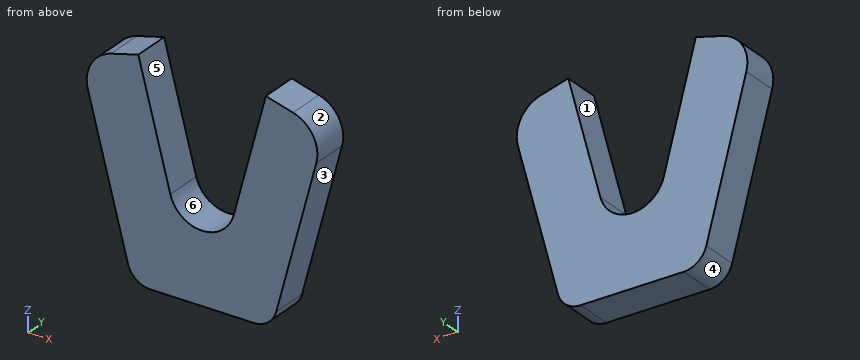
from build123d import *

# Parameters (mm, degrees)
F1_DEPTH = 25.4


with BuildPart() as f1:
    # F0 (on Front) → F1 (new body)
    with BuildSketch(Plane.XZ):
        with BuildLine():
            ThreePointArc((-50.266767, -58.054928), (-44.600918, -66.560398), (-34.925, -69.85))
            Line((-34.925, -69.85), (34.925, -69.85))
            ThreePointArc((34.925, -69.85), (44.600918, -66.560398), (50.266767, -58.054928))
            Line((50.266767, -58.054928), (77.358474, 43.8181))
            ThreePointArc((77.358474, 43.8181), (75.106497, 60.678651), (61.5919, 71.008474))
            Line((61.5919, 71.008474), (43.183091, 75.904039))
            Line((43.183091, 75.904039), (21.478474, -5.7119))
            ThreePointArc((21.478474, -5.7119), (0, -22.225), (-21.478474, -5.7119))
            Line((-21.478474, -5.7119), (-43.183091, 75.904039))
            Line((-43.183091, 75.904039), (-61.5919, 71.008474))
            ThreePointArc((-61.5919, 71.008474), (-75.106497, 60.678651), (-77.358474, 43.8181))
            Line((-77.358474, 43.8181), (-50.266767, -58.054928))
        make_face()
    extrude(amount=F1_DEPTH)


solid = f1.part
Work out the finished part from the listing and answer in its coordinate system (mm). Face numbers are marked on the shaded views. A direction names the side the tool comes from. Give positions to 0.01 mm unless a question says otherwise; leave off trailing zeros. Write each loop counter-clockwise with the first axis right and the second up, starting at its lowest first coordinate (ties: lowest second). Pieces come first, ordered by that corner, then holes. Notation, with made-up numbers: (48.5, -36) - (64.5, -36) arc R33 cw to (64.5, -8) - close; hole circle Ø9 at (-36, 58.5). An arc over 180 degrees is marked (long way). One line per item, written item: value. Start each with the question number.
1. Consider probe 1 along X at (y, z) = (-22.5, 33.5); probe 2 along X at (y, z) = (-18.75, 62); probe 3 along Z at (x, y) = (6, -9.25). Determine where each line is inside the solid, lowest interval first.
2. For the marked faces 1 and 2, determine the directions among +Z, -Z, +X, -X, +Y, -Y from which every point of the face is accessible in a straight line to the end or side of a thin tool.
3. Find section D-D (z = 26.5). Write down the section's boundary in (x, y).
4. Find section B-B (z = -17). Write down the section's boundary in (x, y).
5. Find section A-A (y = -3.5). Write down the section's boundary in (x, z) (3 decimals).
6. For a pull along X with two mould halves and no side action, classify the marked faces 3, 4, 5 and 6 as +X half, -X half, draft (parallel to the pull), parting line (faces both ways), or undercut.
7. Find section C-C (x = -4.5). Write down the section's boundary in (y, z), then the cut area to 3 significant figures.
8. Given pin 1 (3 mm diameter, centred on x = -17.5, y = -15, fed in from +Z); pin 2 (4 mm diameter, centred on y = -20.5, z = -31, fed in from +X), each flat-ended and moving along its own axis, determine where each tip first touches the part or whether it passes through.
Geometry results:
1. probe 1: -74.61 to -31.91, 31.91 to 74.61
1. probe 2: -74.28 to -39.49, 39.49 to 74.28
1. probe 3: -69.85 to -21.4
2. face 1: +Z, +Y, -Y
2. face 2: +X, +Y, -Y
3. outline: (-72.75, -25.4) - (-30.04, -25.4) - (-30.04, 0) - (-72.75, 0) - close; (30.04, -25.4) - (72.75, -25.4) - (72.75, 0) - (30.04, 0) - close
4. outline: (-61.18, -25.4) - (-14.32, -25.4) - (-14.32, 0) - (-61.18, 0) - close; (14.32, -25.4) - (61.18, -25.4) - (61.18, 0) - (14.32, 0) - close
5. outline: (-77.358, 43.818) - (-50.267, -58.055) arc R15.875 ccw to (-34.925, -69.85) - (34.925, -69.85) arc R15.875 ccw to (50.267, -58.055) - (77.358, 43.818) arc R22.225 ccw to (61.592, 71.008) - (43.183, 75.904) - (21.478, -5.712) arc R22.225 cw to (-21.478, -5.712) - (-43.183, 75.904) - (-61.592, 71.008) arc R22.225 ccw to start
6. face 3: +X half
6. face 4: -X half
6. face 5: undercut
6. face 6: undercut
7. outline: (-25.4, -69.85) - (0, -69.85) - (0, -21.76) - (-25.4, -21.76) - close
7. area: 1,220 mm2
8. pin 1: z = -11.53
8. pin 2: x = 57.99
